Job drawing, mm, ordinate dimensions from the low corner. One solid piece. A direction names the side the tool comes from. Give positions to 0.01 mm unless a question says otherwise; leave off trailing zeros. Write each loop counter-clockwise with the first axis right and the second up, starting at its lowest first coordinate (ties: lowest second). Pieces come first, ordered by that corner, then holes. Notation, with made-up numbers: M 64,60.5 L 98,60.5 A14 ccw 98,72.5 Z; hole C 26,47 d9. An arc over 180 degrees is marked long. Answer as CSV lines item,"result". Start each with the question number.
Item 1: Pin check, flat tips, straight feed: pin 1 (3 mm diameter, centred on x = 44, z = 13, fed in from +Y); pin 2 (1.5 mm diameter, centred on y = 26, z = 10.5, fed in from -X); pin 3 (9 mm diameter, centred on y = 27.8, z = 9.5, fed in from +X). Stop position of each tip, or through.
Item 2: 3-axis set-ups, long thin cutter, end or side, ignore diameter. For the marked faces 5, 6 and 7: which of +Z, -Z, +X, -X, +Y, -Y reach the whole face in a straight line?
Item 3: Band-saw the part on A-A, the plane y = 45. List the corners of the cut face in (x, z).
Item 4: Two-plate mould, pull along Y, no slides. Class the marked faces 1, 2, 3 and 4: +Y half, -Y half, draft (parallel to the pull), parting line (faces both ways), or undercut.
Item 5: Wall check: L1, parallel to X at y = 22, z = 14.5; L2, parallel to Z at x = 9.5, y = 28; L3, parallel to X at y = 47, z = 11.25. Give the ranges that are in metal, low to high. Write a range as from..to.
Item 6: Band-saw the part on B-B, the plane z = 9.5. List the corners of the cut face in (x, y).
Item 7: Band-saw the part on D-D, the plane x = 50.5. List the corners of the cut face in (y, z).
Item 8: Band-saw the part on C-C, the plane y = 19.5. List the corners of the cut face in (x, z), then the cut area to 3 significant figures.
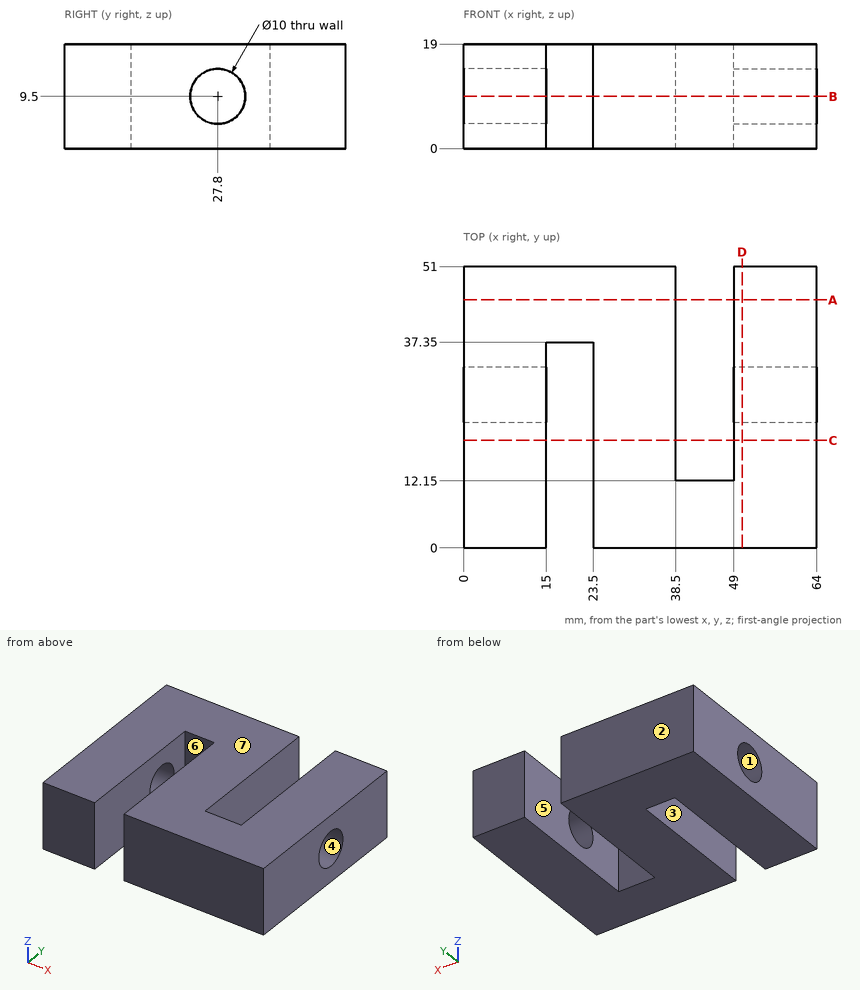
Output:
1,pin 1,"y = 12.15"
1,pin 2,"x = 23.5"
1,pin 3,"x = 38.5"
2,face 5,"+Z, -Z, +Y"
2,face 6,"+Z, -Z, -Y"
2,face 7,"+Z, +X, -X, +Y, -Y"
3,outline,"M 0,0 L 38.5,0 L 38.5,19 L 0,19 Z; M 49,0 L 64,0 L 64,19 L 49,19 Z"
4,face 1,"undercut"
4,face 2,"+Y half"
4,face 3,"draft"
4,face 4,"undercut"
5,L1,"0..15, 23.5..38.5, 49..64"
5,L2,"0..4.5, 14.5..19"
5,L3,"0..38.5, 49..64"
6,outline,"M 0,0 L 15,0 L 15,22.8 L 0,22.8 Z; M 0,32.8 L 15,32.8 L 15,37.35 L 23.5,37.35 L 23.5,0 L 64,0 L 64,22.8 L 49,22.8 L 49,12.15 L 38.5,12.15 L 38.5,51 L 0,51 Z; M 49,32.8 L 64,32.8 L 64,51 L 49,51 Z"
7,outline,"M 0,0 L 51,0 L 51,19 L 0,19 Z; hole C 27.8,9.5 d10"
8,outline,"M 0,0 L 15,0 L 15,19 L 0,19 Z; M 23.5,0 L 38.5,0 L 38.5,19 L 23.5,19 Z; M 49,0 L 64,0 L 64,19 L 49,19 Z"
8,area,"855 mm²"
